Read the model definition and answer for the solid it produces. Units are mm, in the model's axes. Round coordinates to 2 decimals unless told otherwise and drop trailing zeros. Order: outer loops, then holes, each group sorted by start corner. A loop starts at its lowest first (then second) coordinate and runs counter-clockwise, first axis right, second up. Notation, with made-up numbers: (-24, -24.75) - (35, -24.75) arc R28 ccw to (35, 8.25) - close; hole circle Ø1 at (39.5, 36). An arc over 180 degrees is marked (long way). Answer as a JSON object with one key per item and string values. Group by question number.
Q1. A cutting plane is placed at C-C on z = 10. Determine the outline of the cut face in (x, y).
Q2. A cutting plane is placed at D-D on x = 9.5. Determine the outline of the cut face in (y, z).
Q3. A cutting plane is placed at B-B on y = -0.4. Determine the outline of the cut face in (x, z), and give its area (3 significant figures).
Q4. A cutting plane is placed at A-A on z = -5.5. Determine the outline of the cut face in (x, y), and give its area (3 significant figures).
Q5. Consider line 1 (X direction, y = -0.2, z = 8); line 2 (X direction, y = -0.15, z = -9.5); line 3 (X direction, y = -0.1, z = 47.5). Determine where each line is inside the solid, lowest interval first.
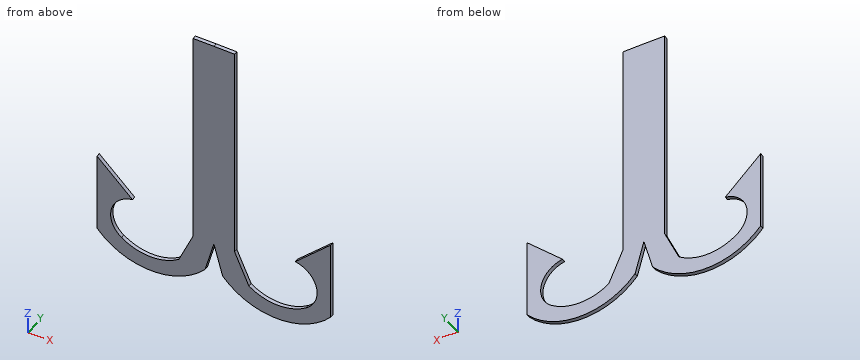
```python
from build123d import *

# Parameters (mm, degrees)
F1_DEPTH = 1.27


with BuildPart() as f1:
    # F0 (on Front) → F1 (new body)
    with BuildSketch(Plane.XZ):
        with BuildLine():
            Line((-2.910425, -10.716616), (0, 0))
            Line((0, 0), (0, 73.787502))
            Line((0, 73.787502), (-6.902514, 73.753235))
            Line((-6.902514, 73.753235), (-6.902514, 0))
            Line((-6.902514, 0), (-11.651456, -10.716616))
            ThreePointArc((-11.651456, -10.716616), (-21.18223, -13.785884), (-30.713003, -10.716616))
            ThreePointArc((-30.713003, -10.716616), (-34.127713, -1.660027), (-27.08658, 4.981095))
            Line((-27.08658, 4.981095), (-38.872454, 16.179355))
            Line((-38.872454, 16.179355), (-38.872454, -10.716616))
            ThreePointArc((-38.872454, -10.716616), (-20.89144, -18.888028), (-2.910425, -10.716616))
        make_face()
        with BuildLine():
            Line((0, 73.787502), (0, 0))
            Line((0, 0), (2.910425, -10.716616))
            ThreePointArc((2.910425, -10.716616), (20.89144, -18.888028), (38.872454, -10.716616))
            Line((38.872454, -10.716616), (38.872454, 16.179355))
            Line((38.872454, 16.179355), (27.08658, 4.981095))
            ThreePointArc((27.08658, 4.981095), (34.127713, -1.660027), (30.713003, -10.716616))
            ThreePointArc((30.713003, -10.716616), (21.18223, -13.785884), (11.651456, -10.716616))
            Line((11.651456, -10.716616), (6.902514, 0))
            Line((6.902514, 0), (6.902514, 73.753235))
            Line((6.902514, 73.753235), (0, 73.787502))
        make_face()
    extrude(amount=F1_DEPTH)


solid = f1.part
```
Result set:
{
 "1": {"outline": "(-38.87, -1.27) - (-32.37, -1.27) - (-32.37, 0) - (-38.87, 0) - close; (-6.9, -1.27) - (6.9, -1.27) - (6.9, 0) - (-6.9, 0) - close; (32.37, -1.27) - (38.87, -1.27) - (38.87, 0) - (32.37, 0) - close"},
 "2": {"outline": "(-1.27, -15.99) - (0, -15.99) - (0, -5.86) - (-1.27, -5.86) - close"},
 "3": {"outline": "(-38.87, -10.72) arc R23.87 ccw to (-2.91, -10.72) - (0, 0) - (2.91, -10.72) arc R23.87 ccw to (38.87, -10.72) - (38.87, 16.18) - (27.09, 4.98) arc R8.73 cw to (30.71, -10.72) arc R16.33 cw to (11.65, -10.72) - (6.9, 0) - (6.9, 73.75) - (0, 73.79) - (-6.9, 73.75) - (-6.9, 0) - (-11.65, -10.72) arc R16.33 cw to (-30.71, -10.72) arc R8.73 cw to (-27.09, 4.98) - (-38.87, 16.18) - close", "area": "1,830 mm²"},
 "4": {"outline": "(-38.87, -1.27) - (-34.15, -1.27) - (-34.15, 0) - (-38.87, 0) - close; (-9.34, -1.27) - (-1.49, -1.27) - (-1.49, 0) - (-9.34, 0) - close; (1.49, -1.27) - (9.34, -1.27) - (9.34, 0) - (1.49, 0) - close; (34.15, -1.27) - (38.87, -1.27) - (38.87, 0) - (34.15, 0) - close", "area": "31.9 mm²"},
 "5": {"line 1": "x = -38.87 to -30.26, -6.9 to 6.9, 30.26 to 38.87", "line 2": "x = -38.87 to -32.08, -11.11 to -2.58, 2.58 to 11.11, 32.08 to 38.87", "line 3": "x = -6.9 to 6.9"}
}
